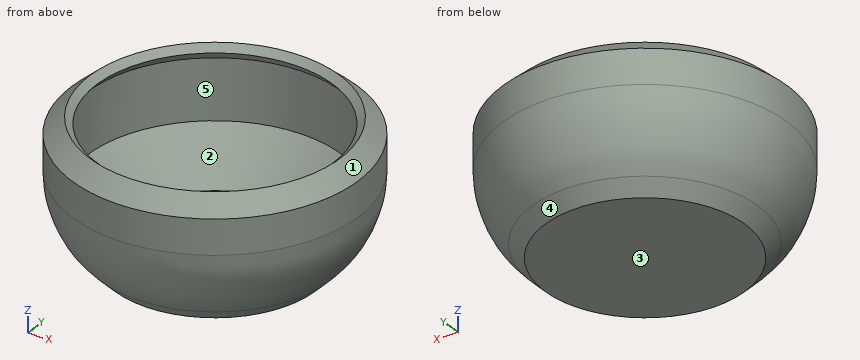
```python
from build123d import *

# Parameters (mm, degrees)
F0_R     = 5
F1_DEPTH = 0.8
F1_TAPER = 45
F4_R     = 5


with BuildPart() as f1:
    # F0 (on Top) → F1 (new body)
    with BuildSketch(Plane.XY):
        Circle(F0_R)
    extrude(amount=F1_DEPTH, taper=F1_TAPER)

    # F2 (on Right) → F3 (revolve)
    with BuildSketch(Plane.YZ):
        Polygon((-7.1213203436, 2.1213203436), (-5, 0), (-4.2, 0.8), (-6.3213203436, 2.9213203436), (-6.3213203436, 5.9213203436), (-5.8819954284, 6.4012245275), (-6.227712161, 6.7177084827), (-7.1213203436, 5.9213203436), align=None)
    revolve(axis=Axis((0, 0, 0.8), (0, 0, -1)))

    # F4
    f4_edges = [f1.edges().sort_by_distance(p)[0] for p in [
        (0, 7.12132, 2.12132),
    ]]
    fillet(f4_edges, radius=F4_R)


solid = f1.part
```
Part model, mm, in its own coordinate system. Face numbers are marked on the shaded views. A direction names the side the tool comes from. Round coordinates to 2 decimals unless told otherwise and drop trailing zeros. Loops run counter-clockwise (first coordinate to the right, second up) from the corner with the lowest first, then second, coordinate; pieces in that order, holes last.
1. Two-plate mould, pull along Y, no slides. Class the marked faces 1, 2 and 3: pulls with the +Y half, pulls with the -Y half, needs draft (parallel to the pull), parting line crosses it, or undercut.
Solutions:
face 1: parting line crosses it
face 2: undercut
face 3: needs draft
2. Slice it at A-A (z = 5). Give the cut face in (x, y).
Solutions:
outline: circle Ø14.24 at (0, 0); hole circle Ø12.64 at (0, 0)
3. Flat gauge pins, fed straight in: pin 1 (4 mm diameter, centred on x = 0.5, y = 5.5, fed in from -Z); pin 2 (1.5 mm diameter, centred on x = 0, z = 1.5, fed in from -Y); pin 3 (4 mm diameter, centred on x = 2.5, z = 3, fed in from -Y); pin 4 (4 mm diameter, centred on x = 1, y = 0, fed in from +Z). Where does each tip first touch, or does it go through?
Solutions:
pin 1: stops at z = 0
pin 2: stops at y = -6.73
pin 3: stops at y = -7.08
pin 4: stops at z = 0.8
4. Drill centre lines: line 1 along Y through (x, z) = (0, 4.55); line 2 along Z through (x, y) = (-3, -1). Where is each one in solid material? Low to high.
Solutions:
line 1: y = -7.12 to -6.32, 6.32 to 7.12
line 2: z = 0 to 0.8
5. 3-axis set-ups, long thin cutter, end or side, ignore diameter. For the marked faces 4 and 5: which of +Z, -Z, +X, -X, +Y, -Y reach the whole face in a straight line?
Solutions:
face 4: -Z
face 5: none
